from build123d import *

# Parameters (mm, degrees)
F0_W     = 3.175
F0_H     = 50.8
F1_DEPTH = 1.5875
F3_DEPTH = 3.176
F5_DEPTH = 3.176
F7_DEPTH = 3.176


with BuildPart() as f1:
    # F0 (on Front) → F1 (new body, symmetric)
    with BuildSketch(Plane.XZ):
        Rectangle(F0_W, F0_H)
    extrude(amount=F1_DEPTH, both=True)

    # F2 (on face) → F3 (cut, through all)
    with BuildSketch(Plane.XZ.offset(1.5875)):
        Polygon((0, 0), (1.5875, 0), (1.5875, 1.5875), align=None)
    extrude(amount=-F3_DEPTH, mode=Mode.SUBTRACT)

    # F4 (on face) → F5 (cut, through all)
    with BuildSketch(Plane.XZ.offset(1.5875)):
        Polygon((1.5875, 0), (0, 0), (1.5875, -1.5875), align=None)
    extrude(amount=-F5_DEPTH, mode=Mode.SUBTRACT)

    # F6 (on face) → F7 (cut, through all)
    with BuildSketch(Plane.XZ.offset(1.5875)):
        Polygon((-1.5875, 18.25625), (-0.80074, 19.05), (-1.5875, 19.84375), align=None)
    extrude(amount=-F7_DEPTH, mode=Mode.SUBTRACT)


solid = f1.part
Verification items for the finished model (mm, model axes). A direction names the side the tool comes from. Give positions to 0.01 mm unless a question says otherwise; leave off trailing zeros. Write each loop counter-clockwise with the first axis right and the second up, starting at its lowest first coordinate (ties: lowest second). Pieces come first, ordered by that corner, then holes.
(1) Cross-section at A-A (x = 0.95). Enter the section's corners in (y, z).
(2) Cross-section at B-B (y = -0.6). Enter the section's corners in (x, z), plus the area to 3 significant figures.
(3) Mould release check, pull along Z, two halves, no side actions. Record for faces 3 (the face through (1.588, 0, 13)), 4 (the face through (0, 0, -25.4)), 5 (the face through (1, 0, -1)), 6 (the face through (0, 0, 25.4)): +Z half, -Z half, draft (parallel to the pull), parting line (faces both ways), or undercut.
(4) Access from +Z, -Z, +X, -X, +Y, -Y to the whole of each face (thin tool, end or side, straight path). Record for faces 1 (the face through (1, 0, 1)), 2 (the face through (-1.588, 0, 23)).
(5) Material ranges on line 1 (Z direction, x = 0.55, y = -0.55); line 2 (Z direction, x = -1.4, y = 1.15); line 3 (X direction, y = -1.4, z = 19), recorded low to high.
Worked out:
1. outline: (-1.59, -25.4) - (1.59, -25.4) - (1.59, -0.95) - (-1.59, -0.95) - close; (-1.59, 0.95) - (1.59, 0.95) - (1.59, 25.4) - (-1.59, 25.4) - close
2. outline: (-1.59, -25.4) - (1.59, -25.4) - (1.59, -1.59) - (0, 0) - (1.59, 1.59) - (1.59, 25.4) - (-1.59, 25.4) - (-1.59, 19.84) - (-0.8, 19.05) - (-1.59, 18.26) - close
2. area: 158 mm2
3. face 3: draft
3. face 4: -Z half
3. face 5: undercut
3. face 6: +Z half
4. face 1: +X, +Y, -Y
4. face 2: +Z, -Z, -X, +Y, -Y
5. line 1: z = -25.4 to -0.55, 0.55 to 25.4
5. line 2: z = -25.4 to 18.45, 19.65 to 25.4
5. line 3: x = -0.85 to 1.59
